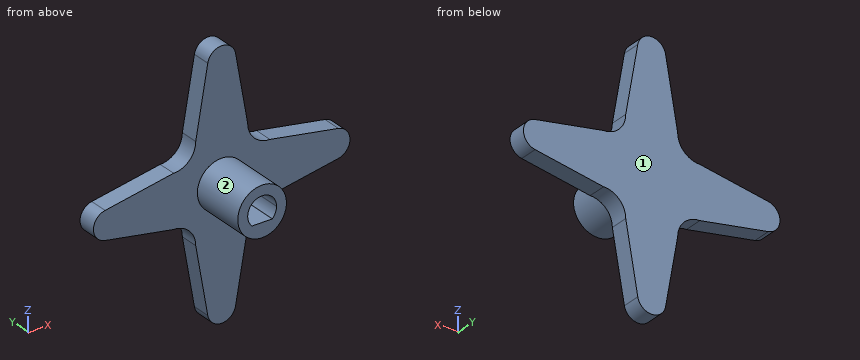
```python
from build123d import *

# Parameters (mm, degrees)
BOSS_EXTRUDE1_DEPTH = 1.325
SKETCH5_R           = 3.5
BOSS_EXTRUDE4_DEPTH = 8
CUT_EXTRUDE1_DEPTH  = 8


with BuildPart() as part:
    # Sketch2 → Boss-Extrude1 (new, symmetric)
    with BuildSketch(Plane(origin=(0, 0, 0), x_dir=(1, 0, 0), z_dir=(0, 1, 0))):
        with BuildLine():
            Line((2, 16.771800738), (3.736481777, 6.923723208))
            ThreePointArc((3.736481777, 6.923723208), (3.979096084, 5.704018717), (4.670003178, 4.670003178))
            ThreePointArc((4.670003178, 4.670003178), (5.704018717, 3.979096084), (6.923723208, 3.736481777))
            Line((6.923723208, 3.736481777), (16.771800738, 2))
            ThreePointArc((16.771800738, 2), (18.45, 0), (16.771800738, -2))
            Line((16.771800738, -2), (6.923723208, -3.736481777))
            ThreePointArc((6.923723208, -3.736481777), (5.704018717, -3.979096084), (4.670003178, -4.670003178))
            ThreePointArc((4.670003178, -4.670003178), (3.979096084, -5.704018717), (3.736481777, -6.923723208))
            Line((3.736481777, -6.923723208), (2, -16.771800738))
            ThreePointArc((2, -16.771800738), (0, -18.45), (-2, -16.771800738))
            Line((-2, -16.771800738), (-3.736481777, -6.923723208))
            ThreePointArc((-3.736481777, -6.923723208), (-3.979096084, -5.704018717), (-4.670003178, -4.670003178))
            ThreePointArc((-4.670003178, -4.670003178), (-5.704018717, -3.979096084), (-6.923723208, -3.736481777))
            Line((-6.923723208, -3.736481777), (-16.771800738, -2))
            ThreePointArc((-16.771800738, -2), (-18.45, 0), (-16.771800738, 2))
            Line((-16.771800738, 2), (-6.923723208, 3.736481777))
            ThreePointArc((-6.923723208, 3.736481777), (-5.704018717, 3.979096084), (-4.670003178, 4.670003178))
            ThreePointArc((-4.670003178, 4.670003178), (-3.979096084, 5.704018717), (-3.736481777, 6.923723208))
            Line((-3.736481777, 6.923723208), (-2, 16.771800738))
            ThreePointArc((-2, 16.771800738), (0, 18.45), (2, 16.771800738))
        make_face()
    extrude(amount=BOSS_EXTRUDE1_DEPTH, both=True)

    # Sketch5 → Boss-Extrude4 (add)
    with BuildSketch(Plane.XZ.offset(1.325)):
        with Locations(Location((0, 0, 0), (0, 0, 90))):
            Circle(SKETCH5_R)
    extrude(amount=BOSS_EXTRUDE4_DEPTH)

    # Sketch6 → Cut-Extrude1 (cut)
    with BuildSketch(Plane.XZ.offset(9.325)):
        with BuildLine():
            ThreePointArc((2.075, 0), (-0.799143979, 1.91493966), (-1.459451952, -1.475))
            Line((-1.459451952, -1.475), (1.459451952, -1.475))
            ThreePointArc((1.459451952, -1.475), (1.91493966, -0.799143979), (2.075, 0))
        make_face()
    extrude(amount=-CUT_EXTRUDE1_DEPTH, mode=Mode.SUBTRACT)


solid = part.part
```
CAD build for the part. Positions are in the model's coordinates, mm. Face numbers are marked on the shaded views. A direction names the side the tool comes from. Coordinates: 2 decimals unless noted, no trailing zeros. Order: outer loops, then holes, each group sorted by start corner. A loop starts at its lowest first (then second) coordinate and runs counter-clockwise, first axis right, second up. Notation, with made-up numbers: M 17.25,-2.75 L 72.25,-2.75 A23 cw 72.25,14.25 Z; hole C 63.25,87.5 d11. An arc over 180 degrees is marked long. Answer as CSV lines item,"result".
1) Drill centre lines: L1, parallel to X at y = -7.5, z = 0 (3 decimals); L2, parallel to Y at x = -1, z = 9 (3 decimals); L3, parallel to X at y = -3, z = -0.5. Where is each one in solid material? Low to high. Write a range as from..to.
Verdict:
L1,"-3.5..-2.075, 2.075..3.5"
L2,"-1.325..1.325"
L3,"-3.46..-2.01, 2.01..3.46"
2) Flat gauge pin, fed straight in: P1, Ø2.5, axis at x = 0.5, y = -4.5, coming from the +Z side. Where does the tip first touch, or does it go through?
Verdict:
P1,"z = 3.5"
3) 3-axis set-ups, long thin cutter, end or side, ignore diameter. For the marked faces 1 and 2: which of +Z, -Z, +X, -X, +Y, -Y reach the whole face in a straight line?
Verdict:
face 1,"+Z, -Z, +X, -X, +Y"
face 2,"-Y"
4) Cut at D-D (x = -12). List the corners of the cut face in (y, z) (3 decimals).
Verdict:
outline,"M -1.325,-2.841 L 1.325,-2.841 L 1.325,2.841 L -1.325,2.841 Z"
5) Cut at A-A (x = 0). List the corners of the cut face in (y, z) (3 decimals).
Verdict:
outline,"M -9.325,-3.5 L -1.325,-3.5 L -1.325,-18.45 L 1.325,-18.45 L 1.325,18.45 L -1.325,18.45 L -1.325,3.5 L -9.325,3.5 L -9.325,2.075 L -1.325,2.075 L -1.325,-1.475 L -9.325,-1.475 Z"
6) Cut at C-C (y = -4). List the corners of the cut face in (x, z) (3 decimals).
Verdict:
outline,"C 0,0 d7; hole M -1.459,-1.475 L 1.459,-1.475 A2.075 ccw long Z"
7) Cut at B-B (z = -2.5). List the corners of the cut face in (x, y) (3 decimals).
Verdict:
outline,"M -13.936,-1.325 L -2.449,-1.325 L -2.449,-9.325 L 2.449,-9.325 L 2.449,-1.325 L 13.936,-1.325 L 13.936,1.325 L -13.936,1.325 Z"
